Geometry: final body of the model. Coordinates: model frame, mm. Face numbers are marked on the shaded views. A direction names the side the tool comes from. Round coordinates to 2 decimals unless told otherwise and drop trailing zeros. Loops run counter-clockwise (first coordinate to the right, second up) from the corner with the lowest first, then second, coordinate; pieces in that order, holes last. Notation, with made-up numbers: (38, 64) - (62, 64) arc R20 cw to (62, 101) - close; hole circle Ø8 at (42.25, 71.25). An arc over 180 degrees is marked (long way). Return JSON: item names as keys, results as strings. Group by question number.
1. Section B-B on y = 24.5. Return loops of the section in (x, z), and give its area (3 significant figures).
2. Set-up query: the marked faces 1, 2, 3, 4 and 5. Return all of +Z, -Z, +X, -X, +Y, -Y with unobstructed straight access to the full face (end or side cutting, diameter ignored); none if empty.
3. Section D-D on x = 4. Return loops of the section in (y, z), and give its area (3 significant figures).
4. Section C-C on z = 6.75. Return loops of the section in (x, y).
5. Section A-A on x = 27.25. Return loops of the section in (y, z).
6. First-contact query: pin 1 Ø4 at (x, z) = (9.5, 5.5) entering from +Y; pin 2 Ø2 at (x, z) = (22.5, 5.5) entering from -Y; pin 3 Ø3 at (x, z) = (8.5, 4.5) entering from -Y. Flat tips, straight axial feed; report the tip coordinate or a pass-through.
7. Material intervals for probe 1 along X at (y, z) = (6.5, 6.5); probe 2 along Y at (x, z) = (27.25, 4.25); probe 3 along Y at (x, z) = (5.5, 5.25), sorted ascending.
8. Draft query along Y for the marked faces 6, 7 and 8. Return one class per face: +Y half, -Y half, draft (parallel to the pull), parting line (faces both ways), or undercut.
from build123d import *

# Parameters (mm, degrees)
BOSS_EXTRUDE1_DEPTH   = 8
FILLET1_R             = 1
FILLET2_R             = 1
FILLET3_R             = 1
CUT_EXTRUDE1_DEPTH    = 7
SKETCH3_R             = 16
CUT_EXTRUDE2_DEPTH    = 7
F_4_0MM_DOWEL_HOLE1_D = 4.5


with BuildPart() as part:
    # Sketch1 → Boss-Extrude1 (new body)
    with BuildSketch(Plane.XY):
        with BuildLine():
            Line((11.013257462, 44.582936616), (7.477723556, 48.118470522))
            ThreePointArc((7.477723556, 48.118470522), (2.881529478, 47.63222476), (3.36777524, 43.036030683))
            Line((3.36777524, 43.036030683), (6.903309146, 39.500496777))
            ThreePointArc((6.903309146, 39.500496777), (6.899494188, 39.494158329), (6.895681204, 39.487818693))
            ThreePointArc((6.895681204, 39.487818693), (1.817587447, 33.297587625), (0, 25.5))
            Line((0, 25.5), (0, 0))
            Line((0, 0), (19, 0))
            Line((19, 0), (19, 4.978942549))
            ThreePointArc((19, 4.978942549), (29.469637429, 3.603949385), (39.500496777, 6.903309146))
            Line((39.500496777, 6.903309146), (43.036030683, 3.36777524))
            ThreePointArc((43.036030683, 3.36777524), (47.63222476, 2.881529478), (48.118470522, 7.477723556))
            Line((48.118470522, 7.477723556), (44.582936616, 11.013257462))
            ThreePointArc((44.582936616, 11.013257462), (44.043786053, 44.043786053), (11.013257462, 44.582936616))
        make_face()
    extrude(amount=BOSS_EXTRUDE1_DEPTH)

    # Fillet1
    # the kernel refuses this fillet: 1 mm, written as the material it adds along each edge
    with BuildSketch(Plane(origin=(6.895681204, 39.487818693, 0), x_dir=(-0.6978515576075072, 0.7162424195373911, 0), z_dir=(0, 0, 1))) as fillet1_piece_1:
        with BuildLine():
            CenterArc((1.091132345, 0.99991544), FILLET1_R, 176.70951396, 94.03559873)
            Line((0.092780983, 1.057313692), (-0.007054153, 1.063053517))
            ThreePointArc((-0.007054153, 1.063053517), (-0.04527045, 0.536700242), (-0.099309015, 0.011735396))
            Line((-0.099309015, 0.011735396), (-0.096713844, -0.025425035))
            ThreePointArc((-0.096713844, -0.025425035), (0.005057841, -0.114302419), (1.105437078, -0.099991544))
            Line((1.105437078, -0.099991544), (1.104136648, 0))
        make_face()
    extrude(amount=8)
    with BuildSketch(Plane(origin=(6.903309146, 39.500496777, 0), x_dir=(-0.7071067811865462, 0.7071067811865487, 0), z_dir=(0, 0, 1))) as fillet1_piece_2:
        with BuildLine():
            CenterArc((1.100472293, 1), FILLET1_R, 175.96440127, 94.03559873)
            Line((0.102951776, 1.070376262), (0.003199724, 1.077413888))
            ThreePointArc((0.003199724, 1.077413888), (-0.102718997, 0.027384376), (-0.097051337, -0.024104732))
            Line((-0.097051337, -0.024104732), (0, -0.1))
            Line((0, -0.1), (1.100472293, -0.1))
            Line((1.100472293, -0.1), (1.100472293, 0))
        make_face()
    extrude(amount=8)

    # Fillet2
    fillet2_edges = [part.edges().sort_by_distance(p)[0] for p in [
        (11.013257462, 44.582936616, 4),
        (44.582936616, 11.013257462, 4),
        (39.500496777, 6.903309146, 4),
    ]]
    fillet(fillet2_edges, radius=FILLET2_R)

    # Fillet3
    fillet3_edges = [part.edges().sort_by_distance(p)[0] for p in [
        (19, 4.978942549, 4),
    ]]
    fillet(fillet3_edges, radius=FILLET3_R)

    # Sketch2 → Cut-Extrude1 (cut)
    with BuildSketch(Plane.XY.offset(8)):
        with BuildLine():
            Line((1, 0), (1, 22.374195455))
            ThreePointArc((1, 22.374195455), (2.695924616, 32.679401027), (9.007717621, 41.000139649))
            ThreePointArc((9.007717621, 41.000139649), (48.848807822, 34.55190705), (20.71331744, 5.616006286))
            ThreePointArc((20.71331744, 5.616006286), (18.805851762, 5.30344249), (18, 3.546534873))
            Line((18, 3.546534873), (18, 0))
            Line((18, 0), (1, 0))
        make_face()
    extrude(amount=-CUT_EXTRUDE1_DEPTH, mode=Mode.SUBTRACT)

    # Sketch3 → Cut-Extrude2 (cut)
    with BuildSketch(Plane.XY.offset(1)):
        with Locations((27.25, 27.406698819)):
            Circle(SKETCH3_R)
    extrude(amount=-CUT_EXTRUDE2_DEPTH, mode=Mode.SUBTRACT)

    # Ø4.0mm Dowel Hole1 (through all)
    with Locations(Plane(origin=(0, 0, 0), x_dir=(-1, 0, 0), z_dir=(0, 0, -1))):
        with Locations((-45.577250602, 5.422749398), (-5.422749398, 45.577250602)):
            Hole(F_4_0MM_DOWEL_HOLE1_D / 2)


solid = part.part
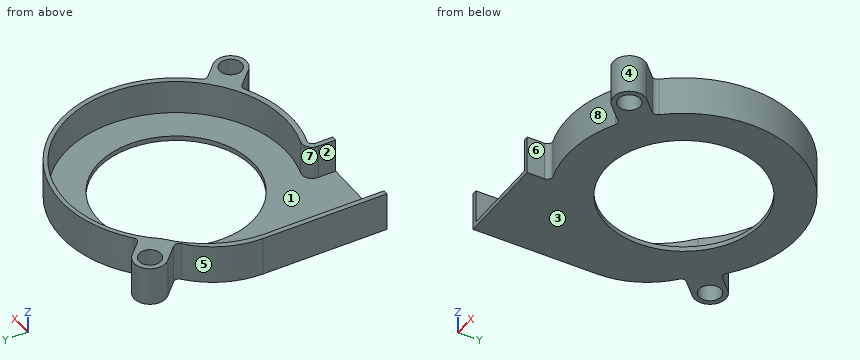
Taken from the geometry:
{
 "1": {"outline": "(0, 0) - (11.52, 0) - (11.52, 1) - (0.93, 1) - (0.93, 8) - (0, 8) - close; (42.98, 0) - (50.84, 0) - (50.84, 8) - (49.81, 8) - (49.81, 1) - (42.98, 1) - close", "area": "33.1 mm2"},
 "2": {"face 1": "+Z", "face 2": "+Z, -Y", "face 3": "-Z, +X, -X, +Y, -Y", "face 4": "+Z, -Z", "face 5": "+Z, -Z, -X"},
 "3": {"outline": "(0, 0) - (36.68, 0) - (36.68, 8) - (35.23, 8) - (35.23, 1) - (0, 1) - close; (42.4, 0) - (43.83, 0) - (43.83, 8) - (42.4, 8) - close; (47.32, 0) - (48.52, 0) - (48.52, 8) - (47.32, 8) - close", "area": "67.9 mm2"},
 "4": {"outline": "(0, 0) - (1, 0) - (1, 22.37) arc R21.71 cw to (9.01, 41) arc R22.75 cw (long way) to (20.71, 5.62) arc R2.06 ccw to (18, 3.55) - (18, 0) - (19, 0) - (19, 3.59) arc R1 cw to (20.29, 4.54) arc R23.75 ccw to (38.85, 6.52) arc R1 cw to (40.04, 6.36) - (43.04, 3.37) arc R3.27 ccw to (48.12, 7.48) - (45.25, 10.34) arc R1 cw to (45.21, 11.7) arc R23.75 ccw to (11.7, 45.21) arc R1 cw to (10.34, 45.25) - (7.48, 48.12) arc R3.27 ccw to (3.37, 43.04) - (6.13, 40.28) arc R1 cw to (6.07, 38.82) arc R17.63 ccw to (0, 25.5) - close; hole circle Ø4.5 at (5.42, 45.58); hole circle Ø4.5 at (45.58, 5.42)"},
 "5": {"outline": "(3.5, 0) - (11.41, 0) - (11.41, 1) - (4.66, 1) - (4.66, 8) - (3.5, 8) - close; (43.41, 0) - (51, 0) - (51, 8) - (50.16, 8) - (50.16, 1) - (43.41, 1) - close"},
 "6": {"pin 1": "y = 48.1", "pin 2": "y = 3.8", "pin 3": "y = 39.16"},
 "7": {"probe 1": "0 to 1, 36.22 to 38.8, 39.87 to 43.6, 47.55 to 48.66", "probe 2": "3.5 to 4.66, 50.16 to 51", "probe 3": "37.43 to 38.3, 40.9 to 43.33, 47.83 to 48.84"},
 "8": {"face 6": "draft", "face 7": "undercut", "face 8": "-Y half"}
}
